```python
from build123d import *

# Parameters (mm, degrees)
EXTRUDE_1_DEPTH = 30
FILLET_2_R      = 3


with BuildPart() as part:
    # 草图1 → 凸台-拉伸1 (new body)
    with BuildSketch(Plane(origin=(0, 0, 0), x_dir=(1, 0, 0), z_dir=(0, 1, 0))):
        with BuildLine():
            Line((-425, 140), (-425, -115))
            Line((-425, -115), (425, -115))
            Line((425, -115), (425, 200))
            Line((425, 200), (-355, 200))
            Line((-355, 200), (-355, 170))
            ThreePointArc((-355, 170), (-360.857864376, 155.857864376), (-375, 150))
            Line((-375, 150), (-415, 150))
            ThreePointArc((-415, 150), (-422.071067812, 147.071067812), (-425, 140))
        make_face()
    extrude(amount=EXTRUDE_1_DEPTH)

    # 圆角2
    fillet_2_edges = [part.edges().sort_by_distance(p)[0] for p in [
        (-360.857864376, 0, -155.857864376),
        (-355, 0, -185),
        (35, 0, -200),
        (425, 0, -42.5),
        (-355, 30, -185),
        (425, 15, 115),
        (-425, 15, 115),
        (-355, 15, -200),
        (425, 15, -200),
        (-360.857864376, 30, -155.857864376),
        (-395, 30, -150),
        (-422.071067812, 30, -147.071067812),
        (-425, 30, -12.5),
        (0, 30, 115),
        (425, 30, -42.5),
        (0, 0, 115),
        (35, 30, -200),
        (-425, 0, -12.5),
        (-422.071067812, 0, -147.071067812),
        (-395, 0, -150),
    ]]
    fillet(fillet_2_edges, radius=FILLET_2_R)


solid = part.part
```
CAD build for the part. Positions are in the model's coordinates, mm. A direction names the side the tool comes from. Round coordinates to 2 decimals unless told otherwise and drop trailing zeros. Use a Markdown table: item, result. Add a question column.
(1) Flat gauge pins, fed straight in: pin 1 (7 mm diameter, centred on y = 9.5, z = -182, fed in from -X); pin 2 (12 mm diameter, centred on x = -401.5, y = 18.5, fed in from -Z). Where does each tip first touch, or does it go through?
(2) Drill centre lines: line 1 (X direction, y = 3.5, z = -182); line 2 (Z direction, x = -381, y = 5.75); line 3 (Z direction, x = -368, y = 7.25) (3 decimals). Where is each one in solid material? Low to high.
(3) Which spindle directions (+Z, -Z, +X, -X, +Y, -Y) get a long thin tool onto all of the face, cutting with end or side? Do faces 1 (the face through (-355, 15, -184)), 2 (the face through (40, 15, -200)). Say none if no direction does.
Geometry says:
| question | item | result |
|---|---|---|
| 1 | pin 1 | stops at x = -355 |
| 1 | pin 2 | stops at z = -150 |
| 2 | line 1 | x = -355 to 425 |
| 2 | line 2 | z = -150 to 115 |
| 2 | line 3 | z = -151.265 to 115 |
| 3 | face 1 | -Z, -X, +Y, -Y |
| 3 | face 2 | -Z, +X, -X, +Y, -Y |
